from build123d import *

# Parameters (mm, degrees)
SKETCH1_W           = 319
SKETCH1_H           = 40
BOSS_EXTRUDE1_DEPTH = 2
SKETCH2_W           = 70
SKETCH2_H           = 8.5
CUT_EXTRUDE1_DEPTH  = 3
SKETCH3_W           = 50
SKETCH3_H           = 8.5
CUT_EXTRUDE2_DEPTH  = 3
FILLET1_R           = 10


with BuildPart() as part:
    # Sketch1 → Boss-Extrude1 (new body)
    with BuildSketch(Plane(origin=(0, 0, 0), x_dir=(1, 0, 0), z_dir=(0, 1, 0))):
        with Locations((159.5, -20)):
            Rectangle(SKETCH1_W, SKETCH1_H)
    extrude(amount=BOSS_EXTRUDE1_DEPTH)

    # Sketch2 → Cut-Extrude1 (cut, through all)
    with BuildSketch(Plane(origin=(0, 2, 0), x_dir=(1, 0, 0), z_dir=(0, 1, 0))):
        with Locations((35, -20)):
            Rectangle(SKETCH2_W, SKETCH2_H)
    cut_extrude1 = extrude(amount=-CUT_EXTRUDE1_DEPTH, mode=Mode.SUBTRACT)

    # Sketch3 → Cut-Extrude2 (cut, through all)
    with BuildSketch(Plane(origin=(0, 2, 0), x_dir=(1, 0, 0), z_dir=(0, 1, 0))):
        with Locations((116.5, -20)):
            Rectangle(SKETCH3_W, SKETCH3_H)
    cut_extrude2 = extrude(amount=-CUT_EXTRUDE2_DEPTH, mode=Mode.SUBTRACT)

    # Mirror1: Cut-Extrude1, Cut-Extrude2 across plane
    add(cut_extrude1.mirror(Plane.ZY.offset(-159.5)), mode=Mode.SUBTRACT)
    add(cut_extrude2.mirror(Plane.ZY.offset(-159.5)), mode=Mode.SUBTRACT)

    # Fillet1
    fillet1_edges = [part.edges().sort_by_distance(p)[0] for p in [
        (0, 1, 0),
        (319, 1, 0),
        (319, 1, 40),
        (0, 1, 40),
    ]]
    fillet(fillet1_edges, radius=FILLET1_R)


solid = part.part
Geometry: final body of the model. Coordinates: model frame, mm. Coordinates: 2 decimals unless noted, no trailing zeros. Order: outer loops, then holes, each group sorted by start corner. A loop starts at its lowest first (then second) coordinate and runs counter-clockwise, first axis right, second up.
1) First-contact query: P1, Ø1, axis at y = 1, z = 18, coming from the +X side; P2, Ø6, axis at x = 134, z = 18, coming from the +Y side; P3, Ø0.6, axis at y = 1, z = 20.5, coming from the -X side. Flat tips, straight axial feed; report the tip coordinate or a pass-through.
Result sheet:
P1: stops at x = 249
P2: stops at y = 2
P3: stops at x = 70
2) Section B-B (x = 129). Return loops of the section in (y, z).
Result sheet:
outline: (0, 0) - (2, 0) - (2, 15.75) - (0, 15.75) - close; (0, 24.25) - (2, 24.25) - (2, 40) - (0, 40) - close
3) Section C-C (y = 0.9). Return loops of the section in (x, z), then the cut area to 3 significant figures.
Result sheet:
outline: (0, 10) arc R10 ccw to (10, 0) - (309, 0) arc R10 ccw to (319, 10) - (319, 15.75) - (249, 15.75) - (249, 24.25) - (319, 24.25) - (319, 30) arc R10 ccw to (309, 40) - (10, 40) arc R10 ccw to (0, 30) - (0, 24.25) - (70, 24.25) - (70, 15.75) - (0, 15.75) - close; hole (91.5, 15.75) - (141.5, 15.75) - (141.5, 24.25) - (91.5, 24.25) - close; hole (177.5, 15.75) - (227.5, 15.75) - (227.5, 24.25) - (177.5, 24.25) - close
area: 10,600 mm2
4) Ray query, probe 1 along X at (y, z) = (1, 19); probe 2 along Z at (x, y) = (57, 0.2); probe 3 along X at (y, z) = (1.35, 37.5). Return the intervals inside material, ascending.
Result sheet:
probe 1: x = 70 to 91.5, 141.5 to 177.5, 227.5 to 249
probe 2: z = 0 to 15.75, 24.25 to 40
probe 3: x = 3.39 to 315.61
5) Section A-A (z = 18.5). Return loops of the section in (x, y).
Result sheet:
outline: (70, 0) - (91.5, 0) - (91.5, 2) - (70, 2) - close; (141.5, 0) - (177.5, 0) - (177.5, 2) - (141.5, 2) - close; (227.5, 0) - (249, 0) - (249, 2) - (227.5, 2) - close
